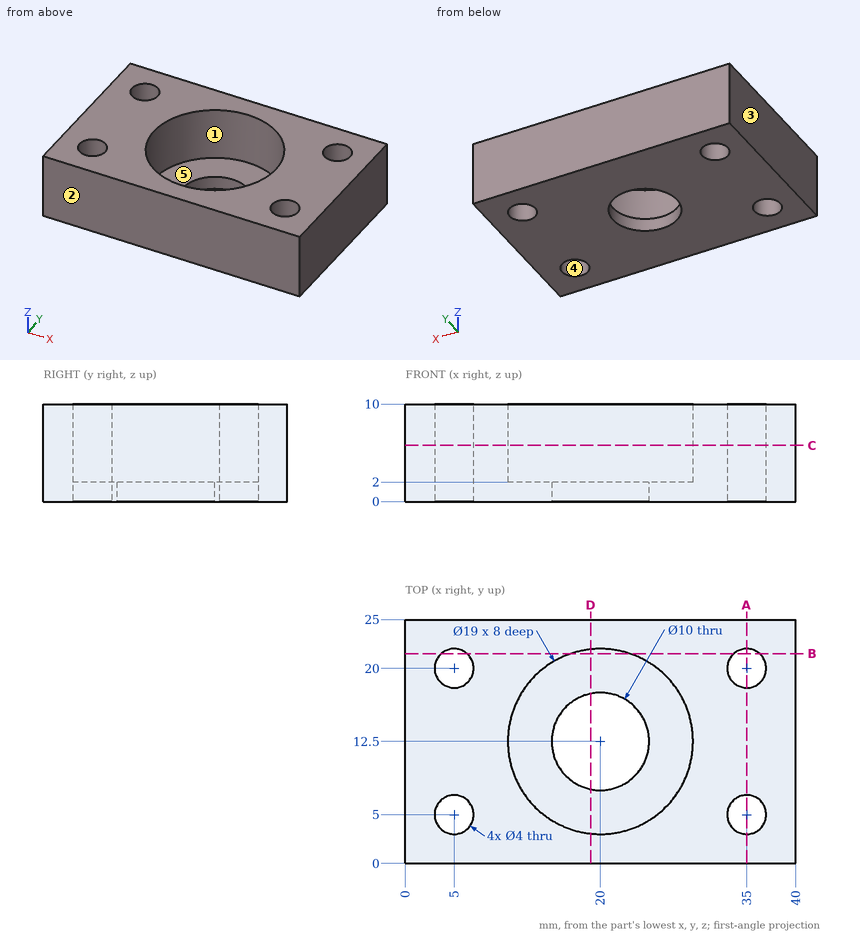
Verification items for this drawing (mm, ordinates from the low corner). A direction names the side the tool comes from. Coordinates: 2 decimals unless noted, no trailing zeros. Write each loop counter-clockwise with the first axis right and the second up, starting at its lowest first coordinate (ties: lowest second). Pieces come first, ordered by that corner, then holes. Notation, with made-up numbers: M 47.5,-5.5 L 97.5,-5.5 A18 ccw 97.5,19.5 Z; hole C 16.25,37 d1. An arc over 180 degrees is marked long. Answer as a JSON object with one key per item and string values.
1. Tool access check on the marked faces 4 and 5. Record the directions out of +Z, -Z, +X, -X, +Y, -Y that give a thin tool (end or side, any length) a straight path to the whole face; none if there is none.
Answers below:
{"face 4": "+Z, -Z", "face 5": "+Z"}
2. Section check C-C, the plane z = 5.75. Enter the section's corners in (x, y).
Answers below:
{"outline": "M 0,0 L 40,0 L 40,25 L 0,25 Z; hole C 5,5 d4; hole C 5,20 d4; hole C 20,12.5 d19; hole C 35,5 d4; hole C 35,20 d4"}
3. Section check D-D, the plane x = 19. Enter the section's corners in (y, z).
Answers below:
{"outline": "M 0,0 L 7.6,0 L 7.6,2 L 3.05,2 L 3.05,10 L 0,10 Z; M 17.4,0 L 25,0 L 25,10 L 21.95,10 L 21.95,2 L 17.4,2 Z"}
4. Section check B-B, the plane y = 21.5. Enter the section's corners in (x, z), plus the area to 3 significant figures.
Answers below:
{"outline": "M 0,0 L 3.68,0 L 3.68,10 L 0,10 Z; M 6.32,0 L 33.68,0 L 33.68,10 L 23.04,10 L 23.04,2 L 16.96,2 L 16.96,10 L 6.32,10 Z; M 36.32,0 L 40,0 L 40,10 L 36.32,10 Z", "area": "298 mm²"}
5. Go/stop test with flat-tipped pins: pin 1 Ø2.5 at (x, y) = (35, 20) entering from -Z; pin 2 Ø4 at (y, z) = (16, 1.5) entering from -X; pin 3 Ø11.5 at (x, y) = (20, 12.5) entering from +Z. Record where each tip stops, or that it passes through.
Answers below:
{"pin 1": "passes through", "pin 2": "stops at x = 0", "pin 3": "stops at z = 2"}
6. Scan lines: L1, parallel to Y at x = 35, z = 7; L2, parallel to Y at x = 20, z = 4; L3, parallel to Y at x = 4.5, z = 3.75. Record each from-to range of solid material in increasing order.
Answers below:
{"L1": "y = 0 to 3, 7 to 18, 22 to 25", "L2": "y = 0 to 3, 22 to 25", "L3": "y = 0 to 3.06, 6.94 to 18.06, 21.94 to 25"}
7. Draft check along X on the marked faces 1, 2 and 3. Enter one of: released by +X, released by -X, zero draft, split by the parting line, or undercut.
Answers below:
{"face 1": "undercut", "face 2": "zero draft", "face 3": "released by -X"}
8. Section check A-A, the plane x = 35. Enter the section's corners in (y, z), plus the area to 3 significant figures.
Answers below:
{"outline": "M 0,0 L 3,0 L 3,10 L 0,10 Z; M 7,0 L 18,0 L 18,10 L 7,10 Z; M 22,0 L 25,0 L 25,10 L 22,10 Z", "area": "170 mm²"}
